from build123d import *

# Parameters (mm, degrees)
SKETCH1_W               = 22.75
SKETCH1_H               = 13.5
BOSS_EXTRUDE1_DEPTH     = 4
FILLET1_SIZE            = 4
CUT_EXTRUDE1_DEPTH      = 2
CUT_EXTRUDE2_DEPTH      = 25.445091674
CUT_EXTRUDE2_DEPTH_BACK = 25.445091674
SKETCH5_W               = 8
SKETCH5_H               = 0.5
SKETCH4_W               = 13.5
SKETCH4_H               = 2
BOSS_EXTRUDE2_DEPTH     = 8
SKETCH6_W               = 4.5
SKETCH6_H               = 10.5
CUT_EXTRUDE3_DEPTH      = 27.529464896
FILLET3_R               = 2


# Some blends are built 0.0001 mm under size
with BuildPart() as part:
    # Sketch1 → Boss-Extrude1 (new body)
    with BuildSketch(Plane(origin=(0, 0, 0), x_dir=(1, 0, 0), z_dir=(0, 1, 0))):
        with Locations((11.375, 6.75)):
            Rectangle(SKETCH1_W, SKETCH1_H)
    extrude(amount=BOSS_EXTRUDE1_DEPTH)

    # Fillet1
    # a fillet whose section is not a circle: 4 mm, written as the material it takes off along each edge
    with BuildSketch(Plane(origin=(22.75, 4, 10), x_dir=(0, -1, 0), z_dir=(0, 0, -1))) as fillet1_piece_1:
        with BuildLine():
            Bezier((FILLET1_SIZE, 0), (0, 0), (0, FILLET1_SIZE), weights=[1, 0.282842712, 1])
            Line((0, FILLET1_SIZE), (0, 0))
            Line((0, 0), (FILLET1_SIZE, 0))
        make_face()
    extrude(amount=33.5, mode=Mode.SUBTRACT)

    # Sketch2 → Cut-Extrude1 (cut)
    with BuildSketch(Plane(origin=(0, 4, 0), x_dir=(1, 0, 0), z_dir=(0, 1, 0))):
        with BuildLine():
            Line((17.75, 0), (17.75, 5.5))
            Line((17.75, 5.5), (2.75, 5.5))
            Line((2.75, 5.5), (2.75, 4.5))
            Line((2.75, 4.5), (10.75, 4.5))
            Line((10.75, 4.5), (10.75, 2.9))
            ThreePointArc((10.75, 2.9), (10.486396103, 2.263603897), (9.85, 2))
            Line((9.85, 2), (9.65, 2))
            ThreePointArc((9.65, 2), (9.013603897, 2.263603897), (8.75, 2.9))
            Line((8.75, 2.9), (8.75, 3))
            Line((8.75, 3), (0, 3))
            Line((0, 3), (0, 0))
            Line((0, 0), (17.75, 0))
        make_face()
        with BuildLine():
            Line((0, 10.5), (0, 13.5))
            Line((0, 13.5), (17.75, 13.5))
            Line((17.75, 13.5), (17.75, 8))
            Line((17.75, 8), (2.75, 8))
            Line((2.75, 8), (2.75, 9))
            Line((2.75, 9), (10.75, 9))
            Line((10.75, 9), (10.75, 10.6))
            ThreePointArc((10.75, 10.6), (10.486396103, 11.236396103), (9.85, 11.5))
            Line((9.85, 11.5), (9.65, 11.5))
            ThreePointArc((9.65, 11.5), (9.013603897, 11.236396103), (8.75, 10.6))
            Line((8.75, 10.6), (8.75, 10.5))
            Line((8.75, 10.5), (0, 10.5))
        make_face()
    extrude(amount=-CUT_EXTRUDE1_DEPTH, mode=Mode.SUBTRACT)

    # Sketch5 → Cut-Extrude2 (cut, two sides: drawn at the far end of the back side and taken through both)
    with BuildSketch(Plane(origin=(0, 0, -8), x_dir=(-1, 0, 0), z_dir=(0, 0, -1)).offset(-CUT_EXTRUDE2_DEPTH_BACK)):
        with Locations((-6.75, 2.25)):
            Rectangle(SKETCH5_W, SKETCH5_H)
    extrude(amount=CUT_EXTRUDE2_DEPTH + CUT_EXTRUDE2_DEPTH_BACK, mode=Mode.SUBTRACT)

    # Sketch4 → Boss-Extrude2 (add)
    with BuildSketch(Plane.ZY):
        with Locations((-6.75, 1)):
            Rectangle(SKETCH4_W, SKETCH4_H)
    extrude(amount=BOSS_EXTRUDE2_DEPTH)

    # Sketch6 → Cut-Extrude3 (cut, through all)
    with BuildSketch(Plane(origin=(0, 2, 0), x_dir=(1, 0, 0), z_dir=(0, 1, 0))):
        with Locations((-4.25, 6.75)):
            Rectangle(SKETCH6_W, SKETCH6_H)
    extrude(amount=-CUT_EXTRUDE3_DEPTH, mode=Mode.SUBTRACT)

    # Fillet3
    fillet3_edges = [part.edges().sort_by_distance(p)[0] for p in [
        (-8, 1, 0),
        (-8, 1, -13.5),
        (-6.5, 1, -12),
        (-6.5, 1, -1.5),
        (0, 2, -6.75),
    ]]
    fillet(fillet3_edges, radius=FILLET3_R - 0.0001)  # a hair under: the kernel refuses the full size


solid = part.part
CAD build for the part. Positions are in the model's coordinates, mm. A direction names the side the tool comes from. Round coordinates to 2 decimals unless told otherwise and drop trailing zeros. Order: outer loops, then holes, each group sorted by start corner. A loop starts at its lowest first (then second) coordinate and runs counter-clockwise, first axis right, second up. Notation, with made-up numbers: (29, 37) -> (50, 37) arc R17 ccw to (50, 47) -> close; hole circle Ø2 at (-37.75, 30.25). An arc over 180 degrees is marked (long way). Write each question's results on one line, items separated by ' | '.
1. Cut at C-C (z = -7.5). Count the separate pieces of the cut face and the enclosed holes in it, plus the area to 3 significant figures.
Findings below:
separate pieces: 2 | enclosed holes: 1 | area: 89.5 mm²
2. Flat gauge pins, fed straight in: P1, Ø0.8, axis at x = 6.5, y = 3, coming from the +Z side; P2, Ø1, axis at y = 3, z = -7.5, coming from the +X side. Where does each tip first touch, or does it go through?
Findings below:
P1: stops at z = -3 | P2: stops at x = 21.13
3. Pull direction X, two halves, no side cores. Call faces 1 (the face through (17.75, 3, -3)), 2 (the face through (-0.6, 2.57, -6.7)), 3 (the face through (-3, 1, -1.5)), 4 (the face through (9, 1, 0)): pulls with the +X half, pulls with the -X half, needs draft (parallel to the pull), parting line crosses it, or undercut.
Findings below:
face 1: undercut | face 2: pulls with the -X half | face 3: undercut | face 4: needs draft
4. Cut at B-B (x = 3.5). Give the cut face in (y, z).
Findings below:
outline: (0, -13.5) -> (2, -13.5) -> (2, 0) -> (0, 0) -> close; (2.5, -10.5) -> (4, -10.5) -> (4, -9) -> (2.5, -9) -> close; (2.5, -8) -> (4, -8) -> (4, -5.5) -> (2.5, -5.5) -> close; (2.5, -4.5) -> (4, -4.5) -> (4, -3) -> (2.5, -3) -> close
5. Wall check: line 1 along Z through (x, y) = (5, 2.8); line 2 along Y through (x, z) = (10, -3.25); line 3 along Z through (x, y) = (9, 2.75). Give the ranges that are in metal, low to high. Write a range as [from, to].
Findings below:
line 1: z = [-10.5, -9], [-8, -5.5], [-4.5, -3] | line 2: y = [0, 2], [2.5, 4] | line 3: z = [-11.22, -9], [-8, -5.5], [-4.5, -2.28]
6. Cut at D-D (x = 12.5). Give the cut face in (y, z), plus the area to 3 significant figures.
Findings below:
outline: (0, -13.5) -> (2, -13.5) -> (2, -8) -> (4, -8) -> (4, -5.5) -> (2, -5.5) -> (2, 0) -> (0, 0) -> close | area: 32.0 mm²
7. 3-axis set-ups, long thin cutter, end or side, ignore diameter. For faces 5 (the face through (9.02, 3.26, -2.26)), 6 (the face through (7, 3, -9)), 7 (the face through (7, 2.5, -4)), 8 (the face through (-5.9, 0.99, -2.07)): which of +Z, -Z, +X, -X, +Y, -Y reach the whole face in a straight line?
Findings below:
face 5: +Z, -X, +Y | face 6: +Y | face 7: +Z, -Z | face 8: +Y, -Y
8. Cut at A-A (x = -4). Give the cut face in (y, z).
Findings below:
outline: (0, -13.5) -> (2, -13.5) -> (2, -12) -> (0, -12) -> close; (0, -1.5) -> (2, -1.5) -> (2, 0) -> (0, 0) -> close
